Work out the finished part from the listing and answer in its coordinate system (mm). Face numbers are marked on the shaded views. A direction names the side the tool comes from. Coordinates: 2 decimals unless noted, no trailing zeros. Write each loop counter-clockwise with the first axis right and the second up, starting at its lowest first coordinate (ties: lowest second). Pieces come first, ordered by that corner, then holes. Notation, with made-up numbers: (-14, 46.25) - (19, 46.25) arc R27 ccw to (19, 76.25) - close; hole circle Ø4 at (41, 31). An arc over 180 degrees is marked (long way). One line per item, written item: value.
```python
from build123d import *

# Parameters (mm, degrees)
SKETCH1_R           = 1.575
BOSS_EXTRUDE1_DEPTH = 3
SKETCH2_W           = 4
SKETCH2_H           = 16
BOSS_EXTRUDE2_DEPTH = 32
SKETCH3_R           = 4.1
CUT_EXTRUDE1_DEPTH  = 35


with BuildPart() as part:
    # Sketch1 → Boss-Extrude1 (new body)
    with BuildSketch(Plane.XY):
        Polygon((0, 0), (0, 32), (9, 32), (9, 20), (19, 20), (19, 32), (28, 32), (28, 0), (19, 0), (19, 12), (9, 12), (9, 0), align=None)
        with Locations((4.5, 27.75)):
            Circle(SKETCH1_R, mode=Mode.SUBTRACT)
        with Locations((4.5, 4.25)):
            Circle(SKETCH1_R, mode=Mode.SUBTRACT)
        with Locations(Location((23.5, 4.25, 0), (0, 0, 180))):
            Circle(SKETCH1_R, mode=Mode.SUBTRACT)
        with Locations(Location((23.5, 27.75, 0), (0, 0, 180))):
            Circle(SKETCH1_R, mode=Mode.SUBTRACT)
    extrude(amount=BOSS_EXTRUDE1_DEPTH)

    # Sketch2 → Boss-Extrude2 (add)
    with BuildSketch(Plane.XY.offset(3)):
        with Locations((7, 16)):
            Rectangle(SKETCH2_W, SKETCH2_H)
        with Locations((21, 16)):
            Rectangle(SKETCH2_W, SKETCH2_H)
    extrude(amount=BOSS_EXTRUDE2_DEPTH)

    # Sketch3 → Cut-Extrude1 (cut)
    with BuildSketch(Plane.ZY.offset(-5)):
        with Locations((21.5, 16)):
            Circle(SKETCH3_R)
    extrude(amount=-CUT_EXTRUDE1_DEPTH, mode=Mode.SUBTRACT)


solid = part.part
```
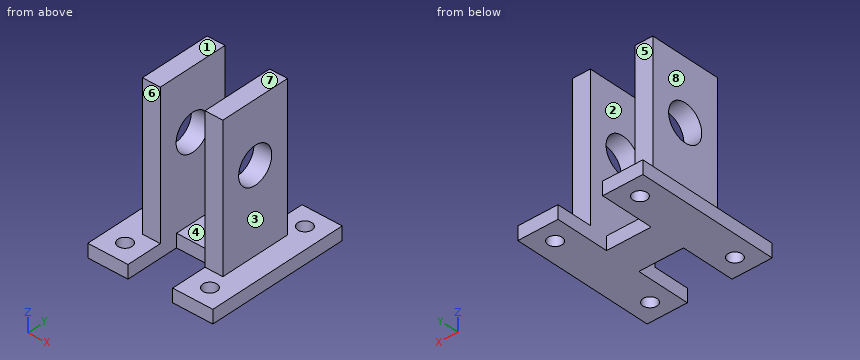
Item 1: Which of the six approach directions +Z, -Z, +X, -X, +Y, -Y give full straight-line access (tool end or side, diameter ignored) to the marked faces 4, 5, 6, 7 and 8?
Evaluation:
face 4: +Z, +Y, -Y
face 5: +Z, +X, -X, +Y
face 6: +Z, +X, -X, -Y
face 7: +Z, +X, -X, +Y, -Y
face 8: +Z, -X, +Y, -Y
Item 2: Section C-C, the plane x = 4.5 is taken. Determine the outline of the cut face in (y, z) (3 decimals), then the cut area to 3 significant figures.
Evaluation:
outline: (0, 0) - (2.675, 0) - (2.675, 3) - (0, 3) - close; (5.825, 0) - (26.175, 0) - (26.175, 3) - (5.825, 3) - close; (29.325, 0) - (32, 0) - (32, 3) - (29.325, 3) - close
area: 77.1 mm2
Item 3: Section D-D, the plane y = 4.25 is taken. Determine the outline of the cut face in (x, z) (3 decimals), then the cut area to 3 significant figures.
Evaluation:
outline: (0, 0) - (2.925, 0) - (2.925, 3) - (0, 3) - close; (6.075, 0) - (9, 0) - (9, 3) - (6.075, 3) - close; (19, 0) - (21.925, 0) - (21.925, 3) - (19, 3) - close; (25.075, 0) - (28, 0) - (28, 3) - (25.075, 3) - close
area: 35.1 mm2
Item 4: Section A-A, the plane z = 27.5 is taken. Determine the outline of the cut face in (x, y), then the cut area to 3 significant figures.
Evaluation:
outline: (5, 8) - (9, 8) - (9, 24) - (5, 24) - close; (19, 8) - (23, 8) - (23, 24) - (19, 24) - close
area: 128 mm2
Item 5: Consider probe 1 along Y at (x, z) = (4.5, 1.5) (3 decimals); probe 2 along Y at (x, z) = (21.05, 21.5); probe 3 along X at (y, z) = (12, 28.5). Determine where each line is inside the solid, lowest interval first.
Evaluation:
probe 1: y = 0 to 2.675, 5.825 to 26.175, 29.325 to 32
probe 2: y = 8 to 11.9, 20.1 to 24
probe 3: x = 5 to 9, 19 to 23
Item 6: Given pin 1 (2.5 mm diameter, centred on x = 23.5, y = 4.25, fed in from +Z); pin 2 (4 mm diameter, centred on y = 23.5, z = 18.5, fed in from +X); pin 3 (6 mm diameter, centred on x = 10.5, y = 4, fed in from -Z); pin 4 (2 mm diameter, centred on x = 18.5, z = 21, fed in from -Y), each flat-ended and moving along its own axis, determine where each tip first touches the part or whether it passes through.
Evaluation:
pin 1: passes through
pin 2: stops at x = 23
pin 3: stops at z = 0
pin 4: stops at y = 8
Item 7: Determine the mould class of the marked faces 1, 2 and 3 for opening direction X: +X half, -X half, draft (parallel to the pull), parting line (faces both ways), or undercut.
Evaluation:
face 1: draft
face 2: undercut
face 3: +X half
Item 8: Section B-B, the plane y = 16 is taken. Determine the outline of the cut face in (x, z).
Evaluation:
outline: (0, 0) - (28, 0) - (28, 3) - (23, 3) - (23, 17.4) - (19, 17.4) - (19, 3) - (9, 3) - (9, 17.4) - (5, 17.4) - (5, 3) - (0, 3) - close; (5, 25.6) - (9, 25.6) - (9, 35) - (5, 35) - close; (19, 25.6) - (23, 25.6) - (23, 35) - (19, 35) - close
